from build123d import *

# Parameters (mm, degrees)
SKETCH3_W               = 149.929020718
SKETCH3_H               = 96.78
SKETCH3_R               = 2.65
BOSS_EXTRUDE1_DEPTH     = 10
SKETCH4_W               = 30
SKETCH4_H               = 12
BOSS_EXTRUDE4_DEPTH     = 13
CUT_EXTRUDE1_DEPTH      = 116.506286536
CUT_EXTRUDE1_DEPTH_BACK = 116.506286536
SKETCH8_R               = 2.65
FILLET1_R               = 1


with BuildPart() as part:
    # Sketch3 → Boss-Extrude1 (new body)
    with BuildSketch(Plane.XY):
        with Locations((-0.035848502, 4.44)):
            Rectangle(SKETCH3_W, SKETCH3_H)
        with Locations((-53.055358861, -17.005)):
            Circle(SKETCH3_R, mode=Mode.SUBTRACT)
        with Locations((-33.055, -17.005)):
            Circle(SKETCH3_R, mode=Mode.SUBTRACT)
        with Locations((33.055, -17.005)):
            Circle(SKETCH3_R, mode=Mode.SUBTRACT)
        with Locations((53.054641139, -17.005)):
            Circle(SKETCH3_R, mode=Mode.SUBTRACT)
        with Locations((-53.055358861, 25.027361408)):
            Circle(SKETCH3_R, mode=Mode.SUBTRACT)
        with Locations((-33.055, 25.027361408)):
            Circle(SKETCH3_R, mode=Mode.SUBTRACT)
        with Locations((-13.055, 24.027361408)):
            Circle(SKETCH3_R, mode=Mode.SUBTRACT)
        with Locations((13.055, 24.027361408)):
            Circle(SKETCH3_R, mode=Mode.SUBTRACT)
        with Locations((33.055, 25.027361408)):
            Circle(SKETCH3_R, mode=Mode.SUBTRACT)
        with Locations((53.054641139, 25.027361408)):
            Circle(SKETCH3_R, mode=Mode.SUBTRACT)
    extrude(amount=BOSS_EXTRUDE1_DEPTH)

    # Sketch4 → Boss-Extrude4 (add)
    with BuildSketch(Plane.XY.offset(10)):
        Polygon((-48.055, 40.83), (-33.055, 40.83), (-18.055, 40.83), (-18.055, 52.83), (-48.055, 52.83), align=None)
        with Locations((33.055, 46.83)):
            Rectangle(SKETCH4_W, SKETCH4_H)
        with Locations((-33.055, -37.95)):
            Rectangle(SKETCH4_W, SKETCH4_H)
        with Locations((33.055, -37.95)):
            Rectangle(SKETCH4_W, SKETCH4_H)
    extrude(amount=BOSS_EXTRUDE4_DEPTH)

    # Sketch8 → Cut-Extrude1 (cut, two sides: drawn at the far end of the back side and taken through both)
    with BuildSketch(Plane(origin=(0, -31.95, 0), x_dir=(1, 0, 0), z_dir=(0, 1, 0)).offset(-CUT_EXTRUDE1_DEPTH_BACK)):
        with Locations(Location((-33.055, -16.5, 0), (0, 0, 270))):
            Circle(SKETCH8_R)
        with Locations(Location((33.055, -16.5, 0), (0, 0, 270))):
            Circle(SKETCH8_R)
    extrude(amount=CUT_EXTRUDE1_DEPTH + CUT_EXTRUDE1_DEPTH_BACK, mode=Mode.SUBTRACT)

    # Fillet1
    fillet1_edges = [part.edges().sort_by_distance(p)[0] for p in [
        (-33.055, 40.83, 10),
        (-18.055, 46.83, 10),
        (-48.055, 46.83, 10),
        (33.055, 40.83, 10),
        (48.055, 46.83, 10),
        (18.055, 46.83, 10),
        (-18.055, -37.95, 10),
        (-33.055, -31.95, 10),
        (-48.055, -37.95, 10),
        (48.055, -37.95, 10),
        (33.055, -31.95, 10),
        (18.055, -37.95, 10),
    ]]
    fillet(fillet1_edges, radius=FILLET1_R)


solid = part.part
Check sheet for the modelled part. Datum: model origin and axes. Units: mm. A direction names the side the tool comes from. Give positions to 0.01 mm unless a question says otherwise; leave off trailing zeros. Write each loop counter-clockwise with the first axis right and the second up, starting at its lowest first coordinate (ties: lowest second). Pieces come first, ordered by that corner, then holes. Notation, with made-up numbers: M -13.5,-24 L 44.5,-24 A17 ccw 44.5,9 Z; hole C 4,29.5 d3. An arc over 180 degrees is marked long. Use one line per item in the form item = value.
(1) Depth check by flat-ended pin: P1, Ø13, axis at y = 44.5, z = 18.5, coming from the -X side (3 decimals); P2, Ø1.5, axis at y = 42, z = 17.5, coming from the +X side (3 decimals); P3, Ø1, axis at x = 0.5, y = -28.5, coming from the +Z side. Enter the tip coordinate at first touch or a pass-through.
Answer block:
P1 = -48.055
P2 = 48.055
P3 = 10
(2) Section check C-C on x = -12. Record the boundary of the cut face in (y, z), plus the area to 3 significant figures.
Answer block:
outline = M -43.95,0 L 21.6,0 L 21.6,10 L -43.95,10 Z; M 26.46,0 L 52.83,0 L 52.83,10 L 26.46,10 Z
area = 919 mm2
(3) Material ranges on line 1 along X through (y, z) = (44.5, 16.5) (3 decimals); line 2 along Y through (x, z) = (20, 17.5); line 3 along Z through (x, y) = (3.5, 20), recorded low to high.
Answer block:
line_1 = -48.055 to -35.705, -30.405 to -18.055, 18.055 to 30.405, 35.705 to 48.055
line_2 = -43.95 to -31.95, 40.83 to 52.83
line_3 = 0 to 10
(4) Section check B-B on z = 16.5. State how many separate pieces and enclosed holes the cut face has, plus the area to 3 significant figures.
Answer block:
separate_pieces = 8
enclosed_holes = 0
area = 1,190 mm2
(5) Section check A-A on x = 41. Record the boundary of the cut face in (y, z), plus the area to 3 significant figures.
Answer block:
outline = M -43.95,0 L 52.83,0 L 52.83,23 L 40.83,23 L 40.83,11 A1 cw 39.83,10 L -30.95,10 A1 cw -31.95,11 L -31.95,23 L -43.95,23 Z
area = 1,280 mm2
(6) Draft check along X on faces 1 (the flat face through (-48.055, -38, 17)), 2 (the flat face through (-1, 52.83, 6)), 3 (the cylindrical face through (34.48, 27.26, 4.93)). Enter one of: pulls with the +X half, pulls with the -X half, needs draft (parallel to the pull), parting line crosses it, or undercut.
Answer block:
face_1 = pulls with the -X half
face_2 = needs draft
face_3 = undercut
(7) Tool access check on faces 4 (the flat face through (48.055, -38, 17)), 5 (the flat face through (-18.055, -38, 17)), 6 (the flat face through (33, 40.83, 20)). Record the directions out of +Z, -Z, +X, -X, +Y, -Y that give a thin tool (end or side, any length) a straight path to the whole face; none if there is none.
Answer block:
face_4 = +Z, +X, +Y, -Y
face_5 = +Z, +Y, -Y
face_6 = +Z, +X, -X
(8) Section check D-D on y = 45.5. Record the boundary of the cut face in (x, z) (3 decimals), plus the area to 3 significant figures.
Answer block:
outline = M -75,0 L 74.929,0 L 74.929,10 L 49.055,10 A1 cw 48.055,11 L 48.055,23 L 18.055,23 L 18.055,11 A1 cw 17.055,10 L -17.055,10 A1 cw -18.055,11 L -18.055,23 L -48.055,23 L -48.055,11 A1 cw -49.055,10 L -75,10 Z; hole C -33.055,16.5 d5.3; hole C 33.055,16.5 d5.3
area = 2,240 mm2
